The model under review builds one solid part; all positions refer to its coordinate system, in mm. Face numbers are marked on the shaded views. A direction names the side the tool comes from. Give positions to 0.01 mm unless a question says otherwise; leave off trailing zeros. Order: outer loops, then holes, each group sorted by start corner. A loop starts at its lowest first (then second) coordinate and runs counter-clockwise, first axis right, second up.
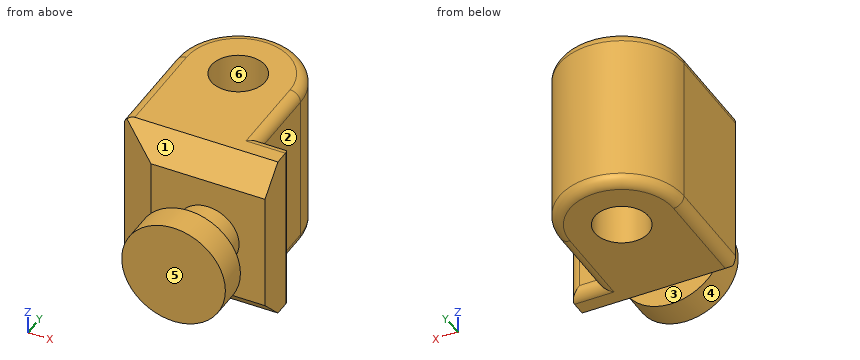
```python
from build123d import *

# Parameters (mm, degrees)
PAD039_DEPTH            = 8.1
SKETCH076_R             = 1.3
POCKET042_DEPTH         = 8.1
POCKET043_DEPTH         = 8
SKETCH078_R             = 1.5
PAD040_DEPTH            = 1.8
SKETCH079_R             = 2.5
PAD041_DEPTH            = 1.4
FILLET024_R             = 0.5
BODY008_PLACEMENT_ANGLE = 270


with BuildPart() as part:
    # Sketch075 → Pad039 (new body)
    with BuildSketch(Plane.XY):
        with BuildLine():
            ThreePointArc((0, 3), (-3, 0), (0, -3))
            Line((0, -3), (4.8, -3))
            Line((4.8, -3), (6, -1.1))
            Line((6, -1.1), (6, 4.4))
            Line((6, 4.4), (3.6, 4.4))
            Line((3.6, 4.4), (3.6, 3))
            Line((3.6, 3), (0, 3))
        make_face()
    extrude(amount=PAD039_DEPTH)

    # Sketch076 (on DatumPlane) → Pocket042 (cut)
    with BuildSketch(Plane.XY.offset(8.1)):
        Circle(SKETCH076_R)
    extrude(amount=-POCKET042_DEPTH, mode=Mode.SUBTRACT)

    # Sketch077 (on DatumPlane) → Pocket043 (cut)
    with BuildSketch(Plane(origin=(0, 4.4, 0), x_dir=(-1, 0, 0), z_dir=(0, 1, 0))):
        Polygon((-4.8, 0), (-6, 1.2), (-6, 0), align=None)
        Polygon((-4.8, 8.1), (-6, 6.9), (-6, 8.1), align=None)
    extrude(amount=-POCKET043_DEPTH, mode=Mode.SUBTRACT)

    # Sketch078 (on DatumPlane) → Pad040 (join)
    with BuildSketch(Plane.YZ.offset(6)):
        with Locations((1.65, 4.05)):
            Circle(SKETCH078_R)
    extrude(amount=PAD040_DEPTH)

    # Sketch079 (on DatumPlane) → Pad041 (join)
    with BuildSketch(Plane.YZ.offset(7.8)):
        with Locations((1.65, 4.05)):
            Circle(SKETCH079_R)
    extrude(amount=PAD041_DEPTH)

    # Fillet024
    fillet024_edges = [part.edges().sort_by_distance(p)[0] for p in [
        (1.8, 3, 8.1),
        (3.6, 3.7, 8.1),
        (3.6, 4.4, 4.05),
        (-3, 0, 8.1),
        (-3, 0, 0),
        (1.8, 3, 0),
        (3.6, 3.7, 0),
        (2.4, -3, 0),
        (2.4, -3, 8.1),
    ]]
    fillet(fillet024_edges, radius=FILLET024_R)


with BuildPart() as part_1:
    # Body008 placement: moved
    add(part.part.moved(Location((31.15, -15, 3.2))).rotate(Axis((31.15, -15, 3.2), (0, 0, 1)), BODY008_PLACEMENT_ANGLE))


solid = part_1.part
```
1. Take a section at D-D (z = 9.5). Write out the cut boundary in (x, y), and give its area (3 significant figures).
2. Take a section at B-B (x = 34.5). Write out the cut boundary in (y, z).
3. Take a section at A-A (z = 7.25). Write out the cut boundary in (x, y), and give its area (3 significant figures).
4. To check wall thickness, follow line 1 (X direction, y = -15, z = 7.5); line 2 (Z direction, x = 32.75, y = -21.5); line 3 (Y direction, x = 31.5, z = 5.25). State the ranges of each line that lie inside material, in increasing order.
5. Insertion check: pin 1 (4 mm diameter, centred on y = -16, z = 7.5, fed in from +X). The pin has a flat end and moves straight along its axis. Give the tip position at first contact, or say it passes through.
6. For the marked faces 1, 2 and 3, list the 3-axis set-ups (+Z, -Z, +X, -X, +Y, -Y) from which the entire face can be reached by the end or side of a thin tool; tool diameter is ignored.
7. Take a section at C-C (y = -16). Write out the cut boundary in (x, z).
8. Draft analysis for pull direction Y (two halves, no side actions). For the marked faces 4, 5 and 6, state which applies: pulls with the +Y half, pulls with the -Y half, needs draft (parallel to the pull), parting line crosses it, or undercut.
Answer:
1. outline: (28.15, -19.8) - (30.05, -21) - (35.55, -21) - (35.55, -19.1) arc R0.5 ccw to (35.05, -18.6) - (34.15, -18.6) - (34.15, -15) arc R3 ccw to (28.15, -15) - close; (31.71, -24.2) - (33.89, -24.2) - (33.89, -22.8) - (31.71, -22.8) - close; hole circle Ø2.6 at (31.15, -15)
1. area: 50.0 mm2
2. outline: (-24.2, 5.42) - (-22.8, 5.42) - (-22.8, 9.08) - (-24.2, 9.08) - close; (-21, 4.4) - (-19.8, 3.2) - (-19.1, 3.2) arc R0.5 ccw to (-18.6, 3.7) - (-18.6, 10.8) arc R0.5 ccw to (-19.1, 11.3) - (-19.8, 11.3) - (-21, 10.1) - close
3. outline: (28.15, -19.8) - (30.05, -21) - (31.3, -21) - (31.3, -22.8) - (30.3, -22.8) - (30.3, -24.2) - (35.3, -24.2) - (35.3, -22.8) - (34.3, -22.8) - (34.3, -21) - (35.55, -21) - (35.55, -19.1) arc R0.5 ccw to (35.05, -18.6) - (34.15, -18.6) - (34.15, -15) arc R3 ccw to (28.15, -15) - close; hole circle Ø2.6 at (31.15, -15)
3. area: 59.4 mm2
4. line 1: x = 28.15 to 29.85, 32.45 to 34.15
4. line 2: z = 5.75 to 8.75
4. line 3: y = -24.2 to -22.8, -21 to -16.25, -13.75 to -12.02
5. pin 1: stops at x = 34.15
6. face 1: +Z, +X, -X, -Y
6. face 2: +Z, -Z, +X, +Y
6. face 3: none
7. outline: (28.15, 3.7) arc R0.5 ccw to (28.65, 3.2) - (30.32, 3.2) - (30.32, 11.3) - (28.65, 11.3) arc R0.5 ccw to (28.15, 10.8) - close; (31.98, 3.2) - (33.65, 3.2) arc R0.5 ccw to (34.15, 3.7) - (34.15, 10.8) arc R0.5 ccw to (33.65, 11.3) - (31.98, 11.3) - close
8. face 4: needs draft
8. face 5: pulls with the -Y half
8. face 6: undercut
